Study the drawing (mm; zero at the part's minimum x, y, z) and answer. Give positions to 0.01 mm unless a question says otherwise; leave off trailing zeros. Write each loop counter-clockwise with the first axis right and the second up, starting at its lowest first coordinate (ties: lowest second). Pieces come first, ordered by that corner, then holes.
1) Find section A-A (y = 12.7). Determine the outline of the cut face in (x, z).
2) Given pin 1 Ø6.5 at (y, z) = (66.5, 9) entering from +X; pin 2 Ø4 at (x, z) = (150, 9.5) entering from -Y; pin 3 Ø5 at (y, z) = (46, 3.5) entering from -X, each flat-ended and moving along its own axis, determine where each tip first touches the part or whether it passes through.
3) Find section C-C (x = 120.65). Determine the outline of the cut face in (y, z), plus the area to 3 significant figures.
4) Straight lines are drawn through the part: probe 1 along Y at (x, z) = (228.6, 19.5); probe 2 along Y at (x, z) = (226.5, 18.5); probe 3 along X at (y, z) = (107, 20.5). For each, find the intervals that lie inside material, in ascending order.
5) Find section B-B (x = 12.7). Determine the outline of the cut face in (y, z).
6) Find section D-D (x = 161). Determine the outline of the cut face in (y, z), plus the area to 3 significant figures.
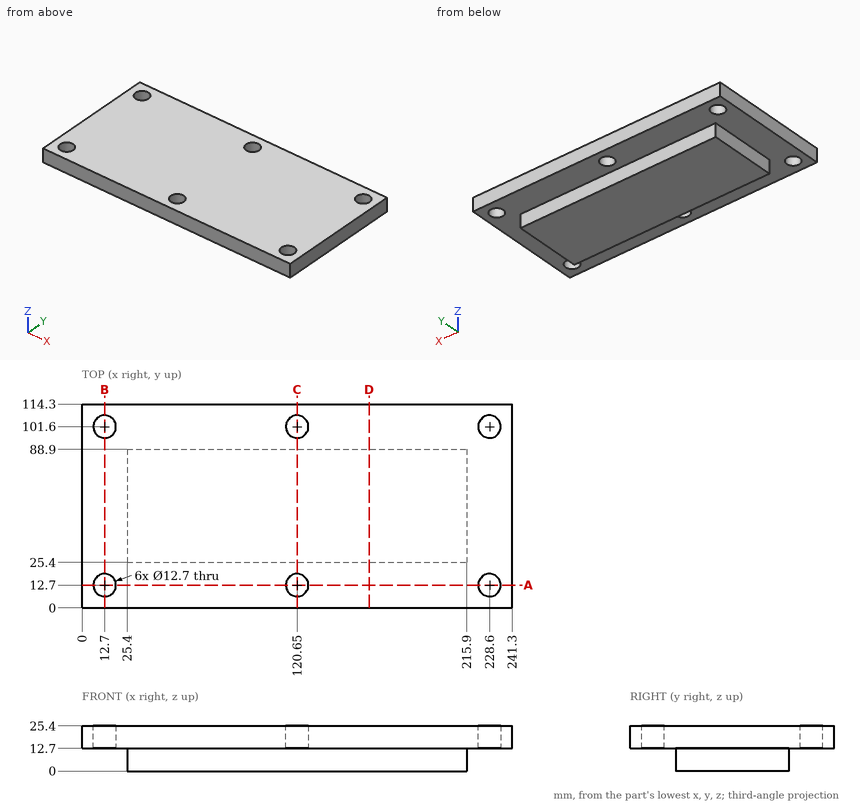
Results:
1. outline: (0, 12.7) - (6.35, 12.7) - (6.35, 25.4) - (0, 25.4) - close; (19.05, 12.7) - (114.3, 12.7) - (114.3, 25.4) - (19.05, 25.4) - close; (127, 12.7) - (222.25, 12.7) - (222.25, 25.4) - (127, 25.4) - close; (234.95, 12.7) - (241.3, 12.7) - (241.3, 25.4) - (234.95, 25.4) - close
2. pin 1: stops at x = 215.9
2. pin 2: stops at y = 25.4
2. pin 3: stops at x = 25.4
3. outline: (0, 12.7) - (6.35, 12.7) - (6.35, 25.4) - (0, 25.4) - close; (19.05, 12.7) - (25.4, 12.7) - (25.4, 0) - (88.9, 0) - (88.9, 12.7) - (95.25, 12.7) - (95.25, 25.4) - (19.05, 25.4) - close; (107.95, 12.7) - (114.3, 12.7) - (114.3, 25.4) - (107.95, 25.4) - close
3. area: 1,940 mm2
4. probe 1: y = 0 to 6.35, 19.05 to 95.25, 107.95 to 114.3
4. probe 2: y = 0 to 6.71, 18.69 to 95.61, 107.59 to 114.3
4. probe 3: x = 0 to 9.36, 16.04 to 117.31, 123.99 to 225.26, 231.94 to 241.3
5. outline: (0, 12.7) - (6.35, 12.7) - (6.35, 25.4) - (0, 25.4) - close; (19.05, 12.7) - (95.25, 12.7) - (95.25, 25.4) - (19.05, 25.4) - close; (107.95, 12.7) - (114.3, 12.7) - (114.3, 25.4) - (107.95, 25.4) - close
6. outline: (0, 12.7) - (25.4, 12.7) - (25.4, 0) - (88.9, 0) - (88.9, 12.7) - (114.3, 12.7) - (114.3, 25.4) - (0, 25.4) - close
6. area: 2,260 mm2
